```python
from build123d import *

# Parameters (mm, degrees)
ESQUISSE1_W      = 30.8
ESQUISSE1_H      = 12.5
ESQUISSE1_R      = 1.847277142
ESQUISSE1_R_2    = 1.96687405
EXTRUSION1_DEPTH = 1
EXTRUSION2_DEPTH = 6
ESQUISSE3_W      = 19.2
ESQUISSE3_H      = 10
EXTRUSION3_DEPTH = 6
ESQUISSE4_R      = 0.272537765
EXTRUSION4_DEPTH = 4.8
CONG_1_R         = 1
EXTRUSION6_START = 6
ESQUISSE7_R      = 0.272537765
EXTRUSION6_DEPTH = 6


with BuildPart() as part:
    # Esquisse1 → Extrusion1 (new body)
    with BuildSketch(Plane.XY):
        with Locations((15.4, 6.25)):
            Rectangle(ESQUISSE1_W, ESQUISSE1_H)
        with Locations((2.9, 6.25)):
            Circle(ESQUISSE1_R, mode=Mode.SUBTRACT)
        with Locations((27.9, 6.25)):
            Circle(ESQUISSE1_R_2, mode=Mode.SUBTRACT)
    extrude(amount=EXTRUSION1_DEPTH)

    # Esquisse2 → Extrusion2 (add)
    with BuildSketch(Plane.XY.offset(1)):
        with BuildLine():
            Line((7.535876796, 11.292947196), (23.264123204, 11.292947196))
            ThreePointArc((23.264123204, 11.292947196), (24.030167647, 10.935734805), (24.248930957, 10.119299018))
            Line((24.248930957, 10.119299018), (22.961743998, 2.819299018))
            ThreePointArc((22.961743998, 2.819299018), (22.619723854, 2.226902752), (21.976936245, 1.992947196))
            Line((21.976936245, 1.992947196), (8.823063755, 1.992947196))
            ThreePointArc((8.823063755, 1.992947196), (8.180276146, 2.226902752), (7.838256002, 2.819299018))
            Line((7.838256002, 2.819299018), (6.551069043, 10.119299018))
            ThreePointArc((6.551069043, 10.119299018), (6.769832353, 10.935734805), (7.535876796, 11.292947196))
        make_face()
        with BuildLine():
            Line((8.131753593, 10.792947196), (22.668246407, 10.792947196))
            ThreePointArc((22.668246407, 10.792947196), (23.434290851, 10.435734805), (23.65305416, 9.619299018))
            Line((23.65305416, 9.619299018), (22.542194182, 3.319299018))
            ThreePointArc((22.542194182, 3.319299018), (22.200174039, 2.726902752), (21.557386429, 2.492947196))
            Line((21.557386429, 2.492947196), (9.242613571, 2.492947196))
            ThreePointArc((9.242613571, 2.492947196), (8.599825961, 2.726902752), (8.257805818, 3.319299018))
            Line((8.257805818, 3.319299018), (7.14694584, 9.619299018))
            ThreePointArc((7.14694584, 9.619299018), (7.365709149, 10.435734805), (8.131753593, 10.792947196))
        make_face(mode=Mode.SUBTRACT)
    extrude(amount=EXTRUSION2_DEPTH)

    # Esquisse3 → Extrusion3 (add)
    with BuildSketch(Plane(origin=(0, 0, 0), x_dir=(-1, 0, 0), z_dir=(0, 0, -1))):
        with Locations((-15.4, 6.25)):
            Rectangle(ESQUISSE3_W, ESQUISSE3_H)
    extrude(amount=EXTRUSION3_DEPTH)

    # Esquisse4 → Extrusion4 (add)
    with BuildSketch(Plane(origin=(0, 0, -6), x_dir=(-1, 0, 0), z_dir=(0, 0, -1))):
        with Locations((-19.98, 8.23)):
            Circle(ESQUISSE4_R)
        with Locations((-17.69, 8.23)):
            Circle(ESQUISSE4_R)
        with Locations((-15.4, 8.23)):
            Circle(ESQUISSE4_R)
        with Locations((-13.11, 8.23)):
            Circle(ESQUISSE4_R)
        with Locations((-10.82, 8.23)):
            Circle(ESQUISSE4_R)
        with Locations((-9.68, 6.25)):
            Circle(ESQUISSE4_R)
        with Locations((-11.97, 6.25)):
            Circle(ESQUISSE4_R)
        with Locations((-14.149725584, 6.068095869)):
            Circle(ESQUISSE4_R)
        with Locations((-16.529732269, 6.22882427)):
            Circle(ESQUISSE4_R)
        with Locations((-18.84, 6.25)):
            Circle(ESQUISSE4_R)
        with Locations((-19.98, 4.27)):
            Circle(ESQUISSE4_R)
        with Locations((-17.69, 4.27)):
            Circle(ESQUISSE4_R)
        with Locations((-15.4, 4.27)):
            Circle(ESQUISSE4_R)
        with Locations((-13.11, 4.27)):
            Circle(ESQUISSE4_R)
        with Locations((-10.82, 4.27)):
            Circle(ESQUISSE4_R)
    extrude(amount=EXTRUSION4_DEPTH)

    # Congé1
    cong_1_edges = [part.edges().sort_by_distance(p)[0] for p in [
        (25, 11.25, -3),
        (25, 1.25, -3),
        (5.8, 1.25, -3),
        (5.8, 11.25, -3),
        (25, 6.25, -6),
        (15.4, 1.25, -6),
        (5.8, 6.25, -6),
        (15.4, 11.25, -6),
        (0, 12.5, 0.5),
        (30.8, 12.5, 0.5),
        (30.8, 0, 0.5),
        (0, 0, 0.5),
    ]]
    fillet(cong_1_edges, radius=CONG_1_R)

    # Esquisse7 → Extrusion6 (add)
    with BuildSketch(Plane.XY.offset(1).offset(EXTRUSION6_START)):
        with Locations(Location((19.98, 8.23, 0), (0, 0, 180))):
            Circle(ESQUISSE7_R)
        with Locations(Location((17.69, 8.23, 0), (0, 0, 180))):
            Circle(ESQUISSE7_R)
        with Locations(Location((15.4, 8.23, 0), (0, 0, 180))):
            Circle(ESQUISSE7_R)
        with Locations(Location((13.11, 8.23, 0), (0, 0, 180))):
            Circle(ESQUISSE7_R)
        with Locations(Location((10.82, 8.23, 0), (0, 0, 180))):
            Circle(ESQUISSE7_R)
        with Locations(Location((9.68, 6.25, 0), (0, 0, 180))):
            Circle(ESQUISSE7_R)
        with Locations(Location((11.97, 6.25, 0), (0, 0, 180))):
            Circle(ESQUISSE7_R)
        with Locations(Location((14.149725584, 6.068095869, 0), (0, 0, 180))):
            Circle(ESQUISSE7_R)
        with Locations(Location((16.529732269, 6.22882427, 0), (0, 0, 180))):
            Circle(ESQUISSE7_R)
        with Locations(Location((18.84, 6.25, 0), (0, 0, 180))):
            Circle(ESQUISSE7_R)
        with Locations(Location((19.98, 4.27, 0), (0, 0, 180))):
            Circle(ESQUISSE7_R)
        with Locations(Location((17.69, 4.27, 0), (0, 0, 180))):
            Circle(ESQUISSE7_R)
        with Locations(Location((15.4, 4.27, 0), (0, 0, 180))):
            Circle(ESQUISSE7_R)
        with Locations(Location((13.11, 4.27, 0), (0, 0, 180))):
            Circle(ESQUISSE7_R)
        with Locations(Location((10.82, 4.27, 0), (0, 0, 180))):
            Circle(ESQUISSE7_R)
    extrude(amount=-EXTRUSION6_DEPTH)


solid = part.part
```
Part model, mm, in its own coordinate system. A direction names the side the tool comes from. Round coordinates to 2 decimals unless told otherwise and drop trailing zeros. Loops run counter-clockwise (first coordinate to the right, second up) from the corner with the lowest first, then second, coordinate; pieces in that order, holes last.
Item 1: Drop flat-ended pins along their axis: P1, Ø2.5, axis at y = 7, z = -2, coming from the -X side; P2, Ø3, axis at x = 17.5, z = 4.5, coming from the +Y side; P3, Ø3, axis at x = 22.5, z = -2, coming from the +Y side. Give the stop position or say it passes through.
Item 2: Cut at A-A, the plane z = 0.5. Give the cut face in (x, y).
Item 3: Cut at D-D, the plane z = -4. Give the cut face in (x, y).
Item 4: Cut at B-B, the plane x = 27.9. Give the cut face in (y, z), then the cut area to 3 significant figures.
Item 5: Mould opens along X. For faces 5 (the face through (15.2, 12.5, 0.5)), 6 (the face through (0.285, 12.199, 0.507)), 7 (the face through (24.02, 10.95, 3.96)), 8 (the face through (22.208, 2.733, 3.958)) say: +X half, -X half, draft (parallel to the pull), parting line (faces both ways), or undercut.
Item 6: 3-axis set-ups, long thin cutter, end or side, ignore diameter. For faces 1 (the face through (7.36, 10.43, 3.96)), 2 (the face through (15, 1.993, 4)), 3 (the face through (6.101, 10.965, -2.535)), 4 (the face through (22.627, 2.233, 3.958)): which of +Z, -Z, +X, -X, +Y, -Y reach the whole face in a straight line?
Item 7: Drill centre lines: line 1 (Y direction, x = 2.9, z = 0.4); line 2 (Z direction, x = 28, y = 10.25); line 3 (Y direction, x = 19, z = 5.25). Where is each one in solid material? Low to high.
Item 8: Cut at C-C, the plane z = -8.75. State how many separate pieces and enclosed holes the cut face has, then the cut area to 3 significant figures.
A:
1. P1: stops at x = 5.8
1. P2: stops at y = 11.29
1. P3: stops at y = 11.25
2. outline: (0, 1) arc R1 ccw to (1, 0) - (29.8, 0) arc R1 ccw to (30.8, 1) - (30.8, 11.5) arc R1 ccw to (29.8, 12.5) - (1, 12.5) arc R1 ccw to (0, 11.5) - close; hole circle Ø3.69 at (2.9, 6.25); hole circle Ø3.93 at (27.9, 6.25)
3. outline: (5.8, 2.25) arc R1 ccw to (6.8, 1.25) - (24, 1.25) arc R1 ccw to (25, 2.25) - (25, 10.25) arc R1 ccw to (24, 11.25) - (6.8, 11.25) arc R1 ccw to (5.8, 10.25) - close
4. outline: (0, 0) - (4.28, 0) - (4.28, 1) - (0, 1) - close; (8.22, 0) - (12.5, 0) - (12.5, 1) - (8.22, 1) - close
4. area: 8.57 mm2
5. face 5: draft
5. face 6: -X half
5. face 7: +X half
5. face 8: undercut
6. face 1: +Z
6. face 2: +Z, +X, -X, -Y
6. face 3: -Z, -X, +Y
6. face 4: +Z, +X, -Y
7. line 1: y = 0 to 4.4, 8.1 to 12.5
7. line 2: z = 0 to 1
7. line 3: y = 1.99 to 2.49, 6.03 to 6.47, 10.79 to 11.29
8. separate pieces: 15
8. enclosed holes: 0
8. area: 3.50 mm2
